Read the model definition and answer for the solid it produces. Units are mm, in the model's axes. A direction names the side the tool comes from. Round coordinates to 2 decimals unless told otherwise and drop trailing zeros. Loops run counter-clockwise (first coordinate to the right, second up) from the corner with the lowest first, then second, coordinate; pieces in that order, holes last. Notation, with made-up numbers: (33.5, 18) - (42.5, 18) arc R11 cw to (42.5, 29) - close; hole circle Ø5 at (65, 84). An arc over 180 degrees is marked (long way). Use CSV: the item, a comma, the result in double quotes. Start each with the question number.
1. Find section C-C (y = -13). Give the vertices of the cut face in (x, z), and give its area (3 significant figures).
2. Find section D-D (x = 13). Give the vertices of the cut face in (y, z), and give its area (3 significant figures).
3. Determine the mould class of faces 1 (the cylindrical face through (0, 10, 87)), 2 (the cylindrical face through (0, -11, 13)), 3 (the flat face through (13, 0, 77.6)), 4 (the cylindrical face through (0.325, 11.536, 81.544)) for opening direction X: +X half, -X half, draft (parallel to the pull), parting line (faces both ways), or undercut.
4. A tool of negligible diameter and unlimited length cuts with its end or side. For faces 5 (the cylindrical face through (0, -10, 87)), 6 (the flat face through (-9, 0, 87)), 7 (the cylindrical face through (-0.325, -11.536, 81.544)), 8 (the flat face through (-14.6, 0, -3)), from which of +Z, -Z, +X, -X, +Y, -Y can it reach the whole face along a straight path? Write none if from no direction.
5. Consider line 1 along Y through (x, z) = (0, 79.75); line 2 along Z through (x, y) = (-7, 3); line 3 along Z through (x, y) = (-16, -6). Determine where each line is inside the solid, lowest interval first.
6. Find section A-A (x = 0). Give the vertices of the cut face in (y, z), and give its area (3 significant figures).
7. Given pin 1 Ø1 at (x, y) = (-11.5, 14) entering from +Z; pin 2 Ø1 at (x, z) = (-13.5, 81) entering from +Y; pin 3 Ø10 at (x, y) = (-12.5, -14) entering from -Z; pin 4 Ø14.5 at (x, y) = (-3.5, 0.5) entering from +Z, each flat-ended and moving along its own axis, determine where each tip first touches the part or whether it passes through.
8. Find section B-B (z = 20.5). Give the vertices of the cut face in (x, y), and give its area (3 significant figures).
Autodesk Inventor part; units mm, degrees
ref_plane "YZ Plane" through (0, 0, 0) normal (1, 0, 0) x (0, 1, 0)
ref_plane "XZ Plane" through (0, 0, 0) normal (0, 1, 0) x (-1, 0, 0)
ref_plane "XY Plane" through (0, 0, 0) normal (0, 0, 1) x (1, 0, 0)
sketch "Sketch1" plane through (0, 0, 0) normal (0, 0, 1) x (1, 0, 0)
  circle A0 centre (0, 0) radius 18
  dimension "MotorDiameter" = 36
extrude "Extrusion1" add sketch "Sketch1" along normal blind 57.1
sketch "Sketch2" plane through (0, 0, 57.1) normal (0, 0, 1) x (1, 0, 0)
  circle A0 centre (0, 0) radius 16
  dimension "d3" = 32
extrude "Extrusion2" add sketch "Sketch2" along normal blind 28.5
sketch "Sketch3" plane through (0, 0, 85.6) normal (0, 0, 1) x (1, 0, 0)
  line L0 (-9, 4.3589) -> (-9, -4.3589)
  line L1 (9, 4.3589) -> (9, -4.3589)
  arc A0 (9, 4.3589) -> (-9, 4.3589) centre (0, 0) ccw
  arc A1 (-9, -4.3589) -> (9, -4.3589) centre (0, 0) ccw
  circle A2 centre (0, 0) radius 16
  dimension "d7" = 18
  dimension "d8" = 9
  dimension "d9" = 10
  dimension "d10" = 10
extrude "Extrusion3" add sketch "Sketch3" along normal blind 3 contours A0 L1 A1 L0
sketch "Sketch4" plane through (0, 0, 88.6) normal (0, 0, 1) x (1, 0, 0)
  arc A0 (-9, -4.3589) -> (9, -4.3589) centre (0, 0) ccw
  circle A1 centre (0, 0) radius 3
  dimension "d13" = 6
extrude "Extrusion4" add sketch "Sketch4" along normal blind 16.3
sketch "Sketch5" plane through (0, 0, 104.9) normal (0, 0, 1) x (1, 0, 0)
  circle A0 centre (0, 0) radius 3
  line L0 (2.5, 1.6583) -> (2.5, -1.6583)
  dimension "d16" = 2.5
extrude "Extrusion5" cut sketch "Sketch5" against normal blind 12 contours A0 L0 picked at (2.5914, -0.3806)
sketch "Sketch6" plane through (0, 0, 85.6) normal (0, 0, 1) x (1, 0, 0)
  circle A0 centre (0, 0) radius 16
  circle A1 centre (0, 0) radius 13
  line L0 (0, 0) -> (-13, 0)
  line L1 (0, 0) -> (-13, 0)
  dimension "d19" = 26
  dimension "d20" = 0
hole "Hole1" at (-13, 0, 85.6) direction (0, 0, -1) diameter 3 depth 8
pattern_circular "Circular Pattern1" count 4 over 360 about axis through (0, 0, 57.1) along (0, 0, 1) of "Hole1"
thread "Thread1"
thread "Thread2"
thread "Thread3"
thread "Thread4"
sketch "Sketch7" plane through (0, 0, 0) normal (0, 0, -1) x (-1, 0, 0)
  line L0 (-14.6, 1.91) -> (-14, 1.91)
  line L1 (-14, 1.91) -> (-14, -1.91)
  line L2 (-14, -1.91) -> (-14.6, -1.91)
  line L3 (-14.6, -1.91) -> (-14.6, 1.91)
  line L4 (14, 1.91) -> (14.6, 1.91)
  line L5 (14.6, 1.91) -> (14.6, -1.91)
  line L6 (14.6, -1.91) -> (14, -1.91)
  line L7 (14, -1.91) -> (14, 1.91)
  point P0 (0, 0)
  point P1 (-14, 0)
  point P2 (14, 0)
  dimension "d39" = 3.82
  dimension "d40" = 0.6
  dimension "d41" = 3.82
  dimension "d42" = 0.6
  dimension "d43" = 28
  dimension "d44" = 14
extrude "Extrusion6" add sketch "Sketch7" along normal blind 6.7
sketch "Sketch8" plane through (0, 0, 0) normal (1, 0, 0) x (0, 1, 0)
  line L0 (-8, 16) -> (8, 16)
  line L1 (8, 10) -> (-8, 10)
  arc A0 (8, 10) -> (8, 16) centre (8, 13) ccw
  arc A1 (-8, 16) -> (-8, 10) centre (-8, 13) ccw
  line L2 (0, 0) -> (0, -14.3353)
  line L3 (0, 0) -> (-17.7641, 0)
  dimension "VentLength" = 16
  dimension "VentHalfWidth" = 3
  dimension "d49" = 8
  dimension "VentOffsetFromEnd" = 10
extrude "Extrusion7" cut sketch "Sketch8" along normal through all both and the other way through all
equation "\"MotorLength\" = FrontLength + BackLength"
equation "\"VentWidth\" = 2 * VentHalfWidth"
properties part number "IG32P-Motor"
Filled sheet:
1,outline,"(-12.45, 0) - (12.45, 0) - (12.45, 57.1) - (9.33, 57.1) - (9.33, 85.6) - (1.5, 85.6) - (1.5, 77.6) - (-1.5, 77.6) - (-1.5, 85.6) - (-9.33, 85.6) - (-9.33, 57.1) - (-12.45, 57.1) - close"
1,area,"1,930 mm²"
2,outline,"(-12.45, 0) - (12.45, 0) - (12.45, 57.1) - (9.33, 57.1) - (9.33, 85.6) - (1.5, 85.6) - (1.5, 77.6) - (-1.5, 77.6) - (-1.5, 85.6) - (-9.33, 85.6) - (-9.33, 57.1) - (-12.45, 57.1) - close; hole (-8, 10) - (8, 10) arc R3 ccw to (8, 16) - (-8, 16) arc R3 ccw to start"
2,area,"1,810 mm²"
3,face 1,"parting line"
3,face 2,"draft"
3,face 3,"undercut"
3,face 4,"undercut"
4,face 5,"+Z, -Y"
4,face 6,"+Z, -X, +Y, -Y"
4,face 7,"+Z"
4,face 8,"-Z, -X, +Y, -Y"
5,line 1,"y = -16 to -14.5, -11.5 to 11.5, 14.5 to 16"
5,line 2,"z = 0 to 10, 16 to 88.6"
5,line 3,"z = 0 to 10, 16 to 57.1"
6,outline,"(-18, 0) - (18, 0) - (18, 57.1) - (16, 57.1) - (16, 85.6) - (14.5, 85.6) - (14.5, 77.6) - (11.5, 77.6) - (11.5, 85.6) - (10, 85.6) - (10, 88.6) - (3, 88.6) - (3, 104.9) - (-3, 104.9) - (-3, 88.6) - (-10, 88.6) - (-10, 85.6) - (-11.5, 85.6) - (-11.5, 77.6) - (-14.5, 77.6) - (-14.5, 85.6) - (-16, 85.6) - (-16, 57.1) - (-18, 57.1) - close; hole (-8, 10) - (8, 10) arc R3 ccw to (8, 16) - (-8, 16) arc R3 ccw to start"
6,area,"2,950 mm²"
7,pin 1,"stops at z = 57.1"
7,pin 2,"stops at y = 9.33"
7,pin 3,"stops at z = 0"
7,pin 4,"stops at z = 104.9"
8,outline,"circle Ø36 at (0, 0)"
8,area,"1,020 mm²"
